```python
from build123d import *

# Parameters (mm, degrees)
PAD_DEPTH                  = 7.6
PAD_MIRRORED_2_DEPTH       = 7.6
PAD001_DEPTH               = 2
PAD001_MIRRORED002_2_DEPTH = 2
SKETCH002_R                = 1
PAD002_DEPTH               = 4
SKETCH003_R                = 2
POCKET073_DEPTH            = 5
CHAMFER035_SIZE            = 1
CHAMFER036_SIZE            = 1
CHAMFER037_SIZE            = 0.5
CHAMFER038_SIZE            = 1.5


with BuildPart() as part:
    # Sketch → Pad (new body)
    with BuildSketch(Plane.XY):
        with BuildLine():
            ThreePointArc((-47.2, 25.2), (-49.32132, 24.32132), (-50.2, 22.2))
            Line((-50.2, 22.2), (-50.2, 0))
            Line((-52.2, 0), (-50.2, 0))
            Line((-52.2, 22.2), (-52.2, 0))
            ThreePointArc((-47.2, 27.2), (-50.735534, 25.735534), (-52.2, 22.2))
            Line((-47.2, 27.2), (0, 27.2))
            Line((0, 27.2), (0, 25.2))
            Line((-47.2, 25.2), (0, 25.2))
        make_face()
    pad = extrude(amount=PAD_DEPTH)

    # Sketch Mirrored 2 → Pad Mirrored 2 (add)
    with BuildSketch(Plane(origin=(0, 0, 0), x_dir=(-1, 0, 0), z_dir=(0, 0, -1))):
        with BuildLine():
            ThreePointArc((-47.2, 25.2), (-49.32132, 24.32132), (-50.2, 22.2))
            Line((-50.2, 22.2), (-50.2, 0))
            Line((-52.2, 0), (-50.2, 0))
            Line((-52.2, 22.2), (-52.2, 0))
            ThreePointArc((-47.2, 27.2), (-50.735534, 25.735534), (-52.2, 22.2))
            Line((-47.2, 27.2), (0, 27.2))
            Line((0, 27.2), (0, 25.2))
            Line((-47.2, 25.2), (0, 25.2))
        make_face()
    pad_mirrored_2 = extrude(amount=-PAD_MIRRORED_2_DEPTH)

    # Mirrored001: Pad, Pad Mirrored 2 across Sketch H_Axis
    add(pad.mirror(Plane.ZX))
    add(pad_mirrored_2.mirror(Plane.ZX))

    # Sketch001 → Pad001 (join)
    with BuildSketch(Plane.XY):
        with BuildLine():
            ThreePointArc((-47.2, 25.2), (-49.32132, 24.32132), (-50.2, 22.2))
            Line((-50.2, 22.2), (-50.2, 0))
            Line((-50.2, 0), (0, 0))
            Line((0, 0), (0, 25.2))
            Line((-47.2, 25.2), (0, 25.2))
        make_face()
    pad001 = extrude(amount=PAD001_DEPTH)

    # Sketch001 Mirrored002 2 → Pad001 Mirrored002 2 (add)
    with BuildSketch(Plane(origin=(0, 0, 0), x_dir=(-1, 0, 0), z_dir=(0, 0, -1))):
        with BuildLine():
            ThreePointArc((-47.2, 25.2), (-49.32132, 24.32132), (-50.2, 22.2))
            Line((-50.2, 22.2), (-50.2, 0))
            Line((-50.2, 0), (0, 0))
            Line((0, 0), (0, 25.2))
            Line((-47.2, 25.2), (0, 25.2))
        make_face()
    pad001_mirrored002_2 = extrude(amount=-PAD001_MIRRORED002_2_DEPTH)

    # Mirrored003: Pad001, Pad001 Mirrored002 2 across Sketch001 H_Axis
    add(pad001.mirror(Plane.ZX))
    add(pad001_mirrored002_2.mirror(Plane.ZX))

    # Sketch002 (on Face19 of MultiTransform001) → Pad002 (join)
    with BuildSketch(Plane.XY.offset(2)):
        with BuildLine():
            ThreePointArc((50.2, 22.2), (49.32132, 24.32132), (47.2, 25.2))
            Line((47.2, 25.2), (44, 25.2))
            Line((44, 22), (44, 25.2))
            ThreePointArc((44, 22), (44.87868, 19.87868), (47, 19))
            Line((47, 19), (50.2, 19))
            Line((50.2, 22.2), (50.2, 19))
        make_face()
        with Locations((47, 22)):
            Circle(SKETCH002_R, mode=Mode.SUBTRACT)
        with BuildLine():
            ThreePointArc((-41, 22), (-38, 19), (-35, 22))
            Line((-35, 22), (-35, 25.2))
            Line((-41, 25.2), (-35, 25.2))
            Line((-41, 22), (-41, 25.2))
        make_face()
        with Locations((-38, 22)):
            Circle(SKETCH002_R, mode=Mode.SUBTRACT)
    pad002 = extrude(amount=PAD002_DEPTH)

    # Mirrored004: Pad002 across Sketch002 H_Axis
    add(pad002.mirror(Plane(origin=(0, 0, 2), x_dir=(0, 0, 1), z_dir=(0, 1, 0))))

    # Sketch003 (on DatumPlane) → Pocket073 (cut)
    with BuildSketch(Plane.XY.offset(2)):
        with Locations((-40, 15)):
            Circle(SKETCH003_R)
        with Locations((40, 15)):
            Circle(SKETCH003_R)
        with Locations((40, -15)):
            Circle(SKETCH003_R)
        with Locations((-40, -15)):
            Circle(SKETCH003_R)
    extrude(amount=-POCKET073_DEPTH, mode=Mode.SUBTRACT)

    # Chamfer035
    chamfer035_edges = [part.edges().sort_by_distance(p)[0] for p in [
        (-35, 23.6, 6),
        (-35, -23.6, 6),
        (48.6, 19, 6),
        (48.6, -19, 6),
    ]]
    chamfer(chamfer035_edges, length=CHAMFER035_SIZE)

    # Chamfer036
    chamfer036_edges = [part.edges().sort_by_distance(p)[0] for p in [
        (0, -27.2, 7.6),
        (0, -27.2, 0),
    ]]
    chamfer(chamfer036_edges, length=CHAMFER036_SIZE)

    # Chamfer037
    chamfer037_edges = [part.edges().sort_by_distance(p)[0] for p in [
        (-39, 22, 6),
        (-39, -22, 6),
        (46, -22, 6),
        (46, 22, 6),
    ]]
    chamfer(chamfer037_edges, length=CHAMFER037_SIZE)

    # Chamfer038
    chamfer038_edges = [part.edges().sort_by_distance(p)[0] for p in [
        (-42, 15, 2),
        (38, 15, 2),
        (38, -15, 2),
        (-42, -15, 2),
    ]]
    chamfer(chamfer038_edges, length=CHAMFER038_SIZE)


solid = part.part
```
Can you work these out from the model? Positions are in its coordinate system, mm. A direction names the side the tool comes from. Round coordinates to 2 decimals unless told otherwise and drop trailing zeros. Loops run counter-clockwise (first coordinate to the right, second up) from the corner with the lowest first, then second, coordinate; pieces in that order, holes last. Notation, with made-up numbers: M 65,29.5 L 114,29.5 A7 cw 114,42.5 Z; hole C 35,42.5 d1. An arc over 180 degrees is marked long. Answer as a JSON object with one key per item and string values. Group by question number.
Q1. We'd pull the mould along Y, two halves only. Please class faces 1 (the flat face through (-38, 24, 6)), 2 (the conical face through (-50.196, -25.263, 0.285)), 3 (the conical face through (50.263, 25.196, 7.315)): +Y half, -Y half, draft (parallel to the pull), parting line (faces both ways), or undercut.
Q2. Imagine slicing it at B-B, the plane y = -15. Please give me the cut outline in (x, z).
Q3. Please list where these lines run through material, in increasing order: L1, parallel to Y at x = 47, z = 3.3; L2, parallel to X at y = -22, z = 3.4; L3, parallel to X at y = -19, z = 5.25.
Q4. On a 3-axis mill with a long thin cutter (end or side, diameter ignored), from which of +Z, -Z, +X, -X, +Y, -Y can I reach the whole of each face in a straight line? I mean faces 4 (the cylindrical face through (-41.474, -13.648, 0.254)), 5 (the flat face through (49, -19, 3)). Say none if no direction works.
Q5. Imagine slicing it at D-D, the plane x = 3. Please give me the cut outline in (y, z).
Q6. Imagine slicing it at C-C, the plane z = 3.5. Count the separate pieces of the cut face and the enclosed holes in it, then the cut area to 3 significant figures.
Q7. Will these pins go through, and if not, where does the flat tip stop? pin 1 (3 mm diameter, centred on x = -37.5, y = -23.5, fed in from +Z); pin 2 (0.9 mm diameter, centred on x = 49, z = 3.5, fed in from -Y).
Q8. Imagine slicing it at A-A, the plane x = 40. Please give me the cut outline in (y, z), then the cut area to 3 significant figures.
Findings:
{
 "1": {"face 1": "undercut", "face 2": "-Y half", "face 3": "+Y half"},
 "2": {"outline": "M -52.2,1 L -51.2,0 L -42,0 L -42,0.5 L -43.5,2 L -50.2,2 L -50.2,7.6 L -51.2,7.6 L -52.2,6.6 Z; M -38,0 L 38,0 L 38,0.5 L 36.5,2 L -36.5,2 L -38,0.5 Z; M 42,0 L 51.2,0 L 52.2,1 L 52.2,6.6 L 51.2,7.6 L 50.2,7.6 L 50.2,2 L 43.5,2 L 42,0.5 Z"},
 "3": {"L1": "y = -27.2 to -23, -21 to -19, 19 to 21, 23 to 27.2", "L2": "x = -52.2 to -50.2, -41 to -39, -37 to -35, 44 to 46, 48 to 52.2", "L3": "x = -52.2 to -50.2, 50.2 to 52.2"},
 "4": {"face 4": "+Z, -Z", "face 5": "+Z"},
 "5": {"outline": "M -27.2,1 L -26.2,0 L 26.2,0 L 27.2,1 L 27.2,6.6 L 26.2,7.6 L 25.2,7.6 L 25.2,2 L -25.2,2 L -25.2,7.6 L -26.2,7.6 L -27.2,6.6 Z"},
 "6": {"separate pieces": "1", "enclosed holes": "5", "area": "729 mm2"},
 "7": {"pin 1": "stops at z = 6", "pin 2": "stops at y = -27.01"},
 "8": {"outline": "M -27.2,1 L -26.2,0 L -17,0 L -17,0.5 L -18.5,2 L -25.2,2 L -25.2,7.6 L -26.2,7.6 L -27.2,6.6 Z; M -13,0 L 13,0 L 13,0.5 L 11.5,2 L -11.5,2 L -13,0.5 Z; M 17,0 L 26.2,0 L 27.2,1 L 27.2,6.6 L 26.2,7.6 L 25.2,7.6 L 25.2,2 L 18.5,2 L 17,0.5 Z", "area": "109 mm2"}
}
